```python
from build123d import *


with BuildPart() as f1:
    # F0 (on Front) → F1 (revolve)
    with BuildSketch(Plane.XZ):
        Polygon((0, 16.911296), (0, 0), (44.608466, 0), (44.608466, 21.264633), (44.608466, 38.319539), (44.608466, 55.661686), (40.960189, 69.201611), (35.32194, 79.182148), (35.32194, 91.453612), (64.839803, 130.268559), (97.342625, 149.649769), (110.609077, 155.38694), (121.22225, 155.38694), (126.197159, 149.649769), (134.820357, 149.649769), (142.448574, 154.217899), (148.418486, 161.100805), (148.418486, 173.519328), (144.770205, 180.207044), (134.820357, 180.207044), (94.357669, 162.556574), (54.889966, 130.268559), (21.0605, 83.4525), (21.0605, 65.94637), (28.025387, 65.94637), (28.025387, 52.313879), (18.738873, 52.313879), (18.738873, 48.949644), (32.005329, 48.949644), (32.005329, 31.426087), (18.738873, 31.426087), (18.738873, 16.911296), align=None)
    revolve(axis=Axis((22.304233, 0, 0), (-1, 0, 0)))


solid = f1.part
```
Input: part model. Units: mm. Frame: model coordinates. A direction names the side the tool comes from. Round coordinates to 2 decimals unless told otherwise and drop trailing zeros. Loops run counter-clockwise (first coordinate to the right, second up) from the corner with the lowest first, then second, coordinate; pieces in that order, holes last. Notation, with made-up numbers: (22.25, 89) -> (60.25, 89) arc R15 ccw to (60.25, 108) -> close; hole circle Ø9 at (-0.5, -32.5). An arc over 180 degrees is marked (long way). One line per item, written item: value.
(1) Section A-A (x = 78.5). Return the cut outline in (y, z).
Geometry check:
outline: circle Ø299.17 at (0, 0); hole circle Ø276.83 at (0, 0)
(2) Mould query, pull axis Y, two halves, no side actions, for faces 1 (the face through (115.99, 46.674, 148.211)), 2 (the face through (22.703, -83.687, -18.584)), 3 (the face through (0, 0, 0)), 4 (the face through (125.956, -91.229, -118.978)). Classes: pulls with the +Y half, pulls with the -Y half, needs draft (parallel to the pull), parting line crosses it, or undercut.
Geometry check:
face 1: undercut
face 2: parting line crosses it
face 3: needs draft
face 4: undercut
(3) Pin query (flat end, axial travel): pin 1 (3 mm diameter, centred on x = 90.5, z = 74.5, fed in from -Y); pin 2 (2 mm diameter, centred on x = 133.5, y = -142.5, fed in from +Z); pin 3 (3 mm diameter, centred on x = 40, z = -82, fed in from +Y). Return the tip coordinate at first contact, or that it passes through.
Geometry check:
pin 1: y = -142.51
pin 2: z = 110.84
pin 3: y = 76.3
(4) Section B-B (x = 115.5). Return the cut outline in (y, z).
Geometry check:
outline: circle Ø343.56 at (0, 0); hole circle Ø310.77 at (0, 0)
(5) Set-up query: faces 5 (the face through (148.418, -51, -153)), 6 (the face through (9.2, -16.5, -3.7)), 7 (the face through (130.6, -146.1, -32.4)). Return all of +Z, -Z, +X, -X, +Y, -Y with unobstructed straight access to the full face (end or side cutting, diameter ignored); none if empty.
Geometry check:
face 5: +Z, -Z, +X, +Y, -Y
face 6: -X
face 7: +X
(6) Material intervals for line 1 (Y direction, x = 24, z = 0); line 2 (Y direction, x = 29, z = 0); line 3 (Y direction, x = 115.5, z = 0), sorted ascending. Write a range as [from, to].
Geometry check:
line 1: [-87.52, -65.95], [-52.31, -48.95], [-31.43, 31.43], [48.95, 52.31], [65.95, 87.52]
line 2: [-94.44, -48.95], [-31.43, 31.43], [48.95, 94.44]
line 3: [-171.78, -155.39], [155.39, 171.78]
